```python
from build123d import *

# Parameters (mm, degrees)
EXTRUDE_START       = -2
EXTRUDE_1_DEPTH     = 2
EXTRUDE_2_DEPTH     = 1
SKETCH_4_R          = 0.85
CUT_EXTRUDE_1_DEPTH = 10


with BuildPart() as part:
    # 草图1 → 旋转1 (revolve)
    with BuildSketch(Plane.XY, mode=Mode.PRIVATE) as revolve_1_sk:
        Polygon((-2.4, 0), (-3.5, 0), (-3.5, 5), (-2.25, 5), (-2.25, 3.8), (-1.25, 3.8), (-1.25, 2.66), (-2.4, 2.66), align=None)
    revolve(revolve_1_sk.sketch.rotate(Axis((0, 0, 0), (0, 1, 0)), 270), axis=Axis((0, 0, 0), (0, 1, 0)))

    # 草图2 → 凸台-拉伸1 (add)
    with BuildSketch(Plane(origin=(0, 2, 0), x_dir=(-1, 0, 0), z_dir=(0, -1, 0)).offset(EXTRUDE_START)):
        with BuildLine():
            Line((-2.49511241, 16.15625), (-3.493157374, 0.21875))
            ThreePointArc((-3.493157374, 0.21875), (0, 3.5), (3.493157374, 0.21875))
            Line((3.493157374, 0.21875), (2.49511241, 16.15625))
            ThreePointArc((2.49511241, 16.15625), (0, 18.5), (-2.49511241, 16.15625))
        make_face()
    extrude(amount=EXTRUDE_1_DEPTH)

    # 草图3 → 凸台-拉伸2 (add)
    with BuildSketch(Plane(origin=(0, 5, 0), x_dir=(1, 0, 0), z_dir=(0, 1, 0))):
        with BuildLine():
            Line((-3.193743885, 5), (3.193743885, 5))
            Line((3.193743885, 5), (3.493157374, 0.21875))
            ThreePointArc((3.493157374, 0.21875), (0, 3.5), (-3.493157374, 0.21875))
            Line((-3.493157374, 0.21875), (-3.193743885, 5))
        make_face()
    extrude(amount=-EXTRUDE_2_DEPTH)

    # 草图4 → 切除-拉伸1 (cut)
    with BuildSketch(Plane.XZ.offset(-2)):
        with Locations(Location((0, -6, 0), (0, 0, 270))):
            Circle(SKETCH_4_R)
        with Locations(Location((0, -16, 0), (0, 0, 270))):
            Circle(SKETCH_4_R)
        with Locations(Location((0, -13.5, 0), (0, 0, 270))):
            Circle(SKETCH_4_R)
        with Locations(Location((0, -8.5, 0), (0, 0, 270))):
            Circle(SKETCH_4_R)
        with Locations(Location((0, -11, 0), (0, 0, 270))):
            Circle(SKETCH_4_R)
    extrude(amount=-CUT_EXTRUDE_1_DEPTH, mode=Mode.SUBTRACT)


solid = part.part
```
Part model, mm, in its own coordinate system. A direction names the side the tool comes from. Coordinates: 2 decimals unless noted, no trailing zeros. Order: outer loops, then holes, each group sorted by start corner. A loop starts at its lowest first (then second) coordinate and runs counter-clockwise, first axis right, second up. Notation, with made-up numbers: (-15.5, 64) -> (-4.5, 64) arc R26 ccw to (-4.5, 88) -> close; hole circle Ø2 at (28.25, -17). An arc over 180 degrees is marked (long way). Put each result on its own line as item: value. Start each with the question number.
(1) Band-saw the part on B-B (z = 0). Give the cut face in (x, y).
(2) Mould opens along X. For faces 1 (the face through (-0.1, 3, -18.5)), 2 (the face through (-0.326, 2.986, -11.785)), 3 (the face through (0, 5, -3)) say: pulls with the +X half, pulls with the -X half, needs draft (parallel to the pull), parting line crosses it, or undercut.
(3) Pin check, flat tips, straight feed: pin 1 Ø2 at (x, z) = (0, -13.5) entering from +Y; pin 2 Ø1.4 at (x, z) = (0, -6) entering from +Y; pin 3 Ø2.5 at (x, z) = (-0.5, 0) entering from -Y; pin 4 Ø1.3 at (x, z) = (-1, 0.5) entering from +Y. Stop position of each tip, or through.
(4) Which spindle directions (+Z, -Z, +X, -X, +Y, -Y) get a long thin tool onto all of the face, cutting with end or side? Do faces 4 (the face through (0, 4.5, -5)), 5 (the face through (-0.154, 1.979, 3.497)), 6 (the face through (1, 3.8, -1)), 7 (the face through (0.26, 2.99, -6.81)). Say none if no direction does.
(5) Band-saw the part on A-A (y = 3.5). Give the cut face in (x, z).
(6) Band-saw the part on C-C (x = 0). Count the separate pieces of the cut face and the enclosed holes in it, then the cut area to 3 significant figures.
(7) Band-saw the part on D-D (z = -2.75). Give the cut face in (x, y), then the cut area to 3 significant figures.
(8) Probe line 1 along X through (y, z) = (4.2, 0); line 2 along X through (y, z) = (3.1, 0); line 3 along Y through (x, z) = (1, -10). List the from-to ranges inside material, lowest first. Write a range as [from, to].
Determined:
1. outline: (-3.5, 0) -> (-2.4, 0) -> (-2.4, 2.66) -> (-1.25, 2.66) -> (-1.25, 3.8) -> (-2.25, 3.8) -> (-2.25, 5) -> (-3.5, 5) -> close; (1.25, 2.66) -> (2.4, 2.66) -> (2.4, 0) -> (3.5, 0) -> (3.5, 5) -> (2.25, 5) -> (2.25, 3.8) -> (1.25, 3.8) -> close
2. face 1: parting line crosses it
2. face 2: undercut
2. face 3: needs draft
3. pin 1: stops at y = 4
3. pin 2: passes through
3. pin 3: stops at y = 2.66
3. pin 4: stops at y = 3.8
4. face 4: -Z, +X, -X, +Y
4. face 5: -Y
4. face 6: +Y
4. face 7: +Y, -Y
5. outline: (-3.49, -0.22) -> (-2.5, -16.16) arc R2.5 ccw to (2.5, -16.16) -> (3.49, -0.22) arc R3.5 ccw (long way) to start; hole circle Ø2.5 at (0, 0); hole circle Ø1.7 at (0, -16); hole circle Ø1.7 at (0, -13.5); hole circle Ø1.7 at (0, -11); hole circle Ø1.7 at (0, -8.5); hole circle Ø1.7 at (0, -6)
6. separate pieces: 7
6. enclosed holes: 0
6. area: 28.5 mm²
7. outline: (-3.33, 2) -> (-2.17, 2) -> (-2.17, 0) -> (2.17, 0) -> (2.17, 2) -> (3.33, 2) -> (3.33, 5) -> (-3.33, 5) -> close
7. area: 28.7 mm²
8. line 1: x = [-3.5, -2.25], [2.25, 3.5]
8. line 2: x = [-3.5, -1.25], [1.25, 3.5]
8. line 3: y = [2, 4]
